```python
from build123d import *

# Parameters (mm, degrees)
F1_DEPTH = 25.4


with BuildPart() as f1:
    # F0 (on Right) → F1 (new body)
    with BuildSketch(Plane.YZ):
        with BuildLine():
            Line((-76.2, -457.2), (76.2, -457.2))
            Line((76.2, -457.2), (76.2, -406.4))
            Line((76.2, -406.4), (12.7, -406.4))
            Line((12.7, -406.4), (12.7, -387.35))
            Line((12.7, -387.35), (76.2, -387.35))
            Line((76.2, -387.35), (76.2, -247.65))
            Line((76.2, -247.65), (12.7, -247.65))
            Line((12.7, -247.65), (12.7, -228.6))
            Line((12.7, -228.6), (76.2, -228.6))
            Line((76.2, -228.6), (76.2, -88.9))
            Line((76.2, -88.9), (12.7, -88.9))
            Line((12.7, -88.9), (12.7, -69.85))
            Line((12.7, -69.85), (76.2, -69.85))
            Line((76.2, -69.85), (76.2, 69.85))
            Line((76.2, 69.85), (25.4, 69.85))
            Line((25.4, 69.85), (25.4, 88.9))
            Line((25.4, 88.9), (76.2, 88.9))
            Line((76.2, 88.9), (76.2, 228.6))
            Line((76.2, 228.6), (38.1, 228.6))
            Line((38.1, 228.6), (38.1, 247.65))
            Line((38.1, 247.65), (76.2, 247.65))
            Line((76.2, 247.65), (76.2, 457.2))
            add(Edge.make_bspline(
                [(76.2, 457.2), (39.3506912784, 410.1214823851), (-42.0134510054, 306.1710057379), (-64.1105424211, 133.5026752831), (-76.2, 39.0347465873)],
                knots=[0, 0, 0, 0, 0.4528937157, 1, 1, 1, 1], degree=3))
            Line((-76.2, 39.0347465873), (-76.2, -457.2))
        make_face()
    extrude(amount=F1_DEPTH)


solid = f1.part
```
Check sheet for the modelled part. Datum: model origin and axes. Units: mm. A direction names the side the tool comes from. Round coordinates to 2 decimals unless told otherwise and drop trailing zeros.
1) Go/stop test with flat-tipped pins: pin 1 Ø5.5 at (x, z) = (16.5, -240.5) entering from +Y; pin 2 Ø5.5 at (x, z) = (15.5, 238) entering from +Y; pin 3 Ø7.5 at (x, y) = (19, 63) entering from +Z. Record where each tip stops, or that it passes through.
2) Mould release check, pull along Z, two halves, no side actions. Record for faces 3 (the flat face through (13, 76.2, -432)), 4 (the flat face through (13, 45, -88.9)), 5 (the flat face through (13, -1, -457.2)): +Z half, -Z half, draft (parallel to the pull), parting line (faces both ways), or undercut.
3) Section check A-A (y = 59.5). Give the number of separate pieces and of enclosed holes in the cut face, and give its area (3 significant figures).
4) Scan lines: line 1 (Z direction, x = 10.5, y = 42); line 2 (Z direction, x = 8, y = 24); line 3 (Y direction, x = 13.25, z = -245). Record each from-to range of solid material in increasing order.
5) Tool access check on faces 1 (the flat face through (13, 76.2, -318)), 2 (the flat face through (13, 50, 88.9)). Record the directions out of +Z, -Z, +X, -X, +Y, -Y that give a thin tool (end or side, any length) a straight path to the whole face; none if there is none.
Result:
1. pin 1: stops at y = 12.7
1. pin 2: stops at y = 38.1
1. pin 3: stops at z = 445.11
2. face 3: draft
2. face 4: undercut
2. face 5: -Z half
3. separate pieces: 6
3. enclosed holes: 0
3. area: 20,300 mm2
4. line 1: z = -457.2 to -406.4, -387.35 to -247.65, -228.6 to -88.9, -69.85 to 69.85, 88.9 to 228.6, 247.65 to 412.6
4. line 2: z = -457.2 to -406.4, -387.35 to -247.65, -228.6 to -88.9, -69.85 to 387.14
4. line 3: y = -76.2 to 12.7
5. face 1: +Z, -Z, +X, -X, +Y
5. face 2: +X, -X, +Y
